from build123d import *

# Parameters (mm, degrees)
SKETCH011_W     = 40
SKETCH011_H     = 30
PAD003_DEPTH    = 10
CHAMFER_SIZE    = 3
PAD_DEPTH       = 17
POCKET_DEPTH    = 5
POCKET001_DEPTH = 4
POCKET002_DEPTH = 40.001
POCKET003_DEPTH = 40.001
PAD001_DEPTH    = 58
PAD002_DEPTH    = 8
POCKET004_DEPTH = 5
SKETCH010_R     = 3.1
POCKET005_DEPTH = 8.001
SKETCH005_R     = 3.4
POCKET006_DEPTH = 41.001
SKETCH012_R     = 8.1
POCKET007_DEPTH = 58.001
POCKET008_DEPTH = 57.5


with BuildPart() as inner_part:
    # Sketch011 → Pad003 (new body)
    with BuildSketch(Plane.XZ.offset(3.5)):
        with Locations((25, 30)):
            Rectangle(SKETCH011_W, SKETCH011_H)
    extrude(amount=PAD003_DEPTH)

    # Chamfer
    chamfer_edges = [inner_part.edges().sort_by_distance(p)[0] for p in [
        (25, -3.5, 45),
        (25, -13.5, 45),
    ]]
    chamfer(chamfer_edges, length=CHAMFER_SIZE)


with BuildPart() as rod_guide_slot:
    # Sketch → Pad (new body)
    with BuildSketch(Plane.XZ):
        Polygon((0, 0), (0, 13.079746), (-5, 21.74), (-5, 39.8), (0, 39.8), (0, 58), (40, 58), (40, 45), (31.339746, 30), (40, 15), (40, 0), align=None)
    extrude(amount=PAD_DEPTH)

    # Sketch001 → Pocket (cut)
    with BuildSketch(Plane(origin=(-5, 0, 0), x_dir=(0, 0, -1), z_dir=(-1, 0, 0))):
        Polygon((-34.892523, 17), (-39.8, 8.5), (-34.892523, 0), (-42.892523, 0), (-42.892523, 17), align=None)
    extrude(amount=-POCKET_DEPTH, mode=Mode.SUBTRACT)

    # Sketch002 → Pocket001 (cut)
    with BuildSketch(Plane(origin=(-5, 0, 0), x_dir=(0, 0, -1), z_dir=(-1, 0, 0))):
        Polygon((-35.89, 8.5), (-32.945, 13.60089), (-27.055, 13.60089), (-24.11, 8.5), (-27.055, 3.39911), (-32.945, 3.39911), align=None)
    extrude(amount=-POCKET001_DEPTH, mode=Mode.SUBTRACT)

    # Sketch003 → Pocket002 (cut, through all)
    with BuildSketch(Plane(origin=(0, 0, 0), x_dir=(0, 0, -1), z_dir=(-1, 0, 0))):
        with BuildLine():
            Line((-55.51292, 9.75), (-55.51292, 7.25))
            Line((-55.51292, 7.25), (-53.88146, 5.61854))
            ThreePointArc((-53.88146, 5.61854), (-46.925, 8.5), (-53.88146, 11.38146))
            Line((-55.51292, 9.75), (-53.88146, 11.38146))
        make_face()
    extrude(amount=-POCKET002_DEPTH, mode=Mode.SUBTRACT)

    # Sketch004 → Pocket003 (cut, through all)
    with BuildSketch(Plane(origin=(0, 0, 0), x_dir=(0, 0, -1), z_dir=(-1, 0, 0))):
        with BuildLine():
            Line((-10.51292, 9.75), (-10.51292, 7.25))
            Line((-10.51292, 7.25), (-8.88146, 5.61854))
            ThreePointArc((-8.88146, 5.61854), (-1.925, 8.5), (-8.88146, 11.38146))
            Line((-10.51292, 9.75), (-8.88146, 11.38146))
        make_face()
    extrude(amount=-POCKET003_DEPTH, mode=Mode.SUBTRACT)

    # Sketch006 → Pad001 (new body)
    with BuildSketch(Plane(origin=(0, 0, 0), x_dir=(1, 0, 0), z_dir=(0, 0, -1))):
        with BuildLine():
            Line((4, 23.5), (4, 17))
            Line((4, 17), (26, 17))
            Line((26, 23.5), (26, 17))
            ThreePointArc((26, 23.5), (15, 34.5), (4, 23.5))
        make_face()
    extrude(amount=-PAD001_DEPTH)

    # Sketch007 → Pad002 (new body)
    with BuildSketch(Plane(origin=(0, 0, 0), x_dir=(1, 0, 0), z_dir=(0, 0, -1))):
        Polygon((25.63, 17), (25.63, 26.32), (28, 30.43), (36, 30.43), (40, 23.5), (40, 17), align=None)
    extrude(amount=-PAD002_DEPTH)

    # Sketch009 → Pocket004 (cut)
    with BuildSketch(Plane(origin=(0, 0, 8), x_dir=(-1, 0, 0), z_dir=(0, 0, 1))):
        Polygon((-36.601482, 23.5), (-34.300741, 27.485), (-29.699259, 27.485), (-27.398518, 23.5), (-29.699259, 19.515), (-34.300741, 19.515), align=None)
    extrude(amount=-POCKET004_DEPTH, mode=Mode.SUBTRACT)

    # Sketch010 → Pocket005 (cut, through all)
    with BuildSketch(Plane(origin=(0, 0, 8), x_dir=(-1, 0, 0), z_dir=(0, 0, 1))):
        with Locations((-32, 23.5)):
            Circle(SKETCH010_R)
    extrude(amount=-POCKET005_DEPTH, mode=Mode.SUBTRACT)

    # Cut001: cut inner-part
    add(inner_part.part, mode=Mode.SUBTRACT)

    # Sketch005 → Pocket006 (cut, through all)
    with BuildSketch(Plane(origin=(-1, 0, 0), x_dir=(0, -1, 0), z_dir=(-1, 0, 0))):
        with Locations((8.5, 30)):
            Circle(SKETCH005_R)
    extrude(amount=-POCKET006_DEPTH, mode=Mode.SUBTRACT)

    # Sketch012 → Pocket007 (cut, through all)
    with BuildSketch(Plane.XY.offset(58)):
        with Locations((15, -23.5)):
            Circle(SKETCH012_R)
    extrude(amount=-POCKET007_DEPTH, mode=Mode.SUBTRACT)

    # Sketch013 → Pocket008 (cut)
    with BuildSketch(Plane.XY.offset(58)):
        Polygon((22.127646, -25.72736), (25.627646, -26.864579), (25.627646, -27.914579), (22.127646, -26.77736), align=None)
    extrude(amount=-POCKET008_DEPTH, mode=Mode.SUBTRACT)


solid = rod_guide_slot.part
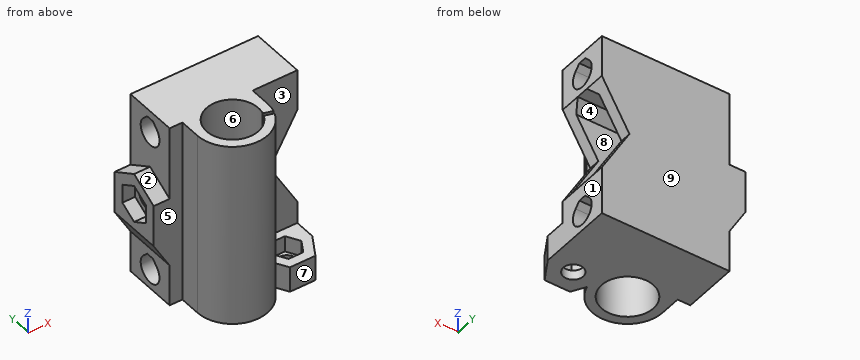
Could you check a few things on this model? Use its own coordinates, in mm. Face numbers are marked on the shaded views. A direction names the side the tool comes from. Round coordinates to 2 decimals unless told otherwise and drop trailing zeros. Write each loop counter-clockwise with the first axis right and the second up, starting at its lowest first coordinate (ties: lowest second). Pieces come first, ordered by that corner, then holes. Notation, with made-up numbers: (28, 45) - (82, 45) arc R28 ccw to (82, 66) - close; hole circle Ø2 at (-35.75, -7.75). An arc over 180 degrees is marked (long way). Use a Markdown table: item, result.
Q1. I want a section at C-C (z = 51). List the corners of the cut face in (x, y) for me (3 decimals), plus the area to 3 significant figures.
Output values:
| item | result |
|---|---|
| outline | (0, -17) - (4, -17) - (4, -23.5) arc R11 ccw to (25.143, -27.757) - (22.372, -26.857) arc R8.1 cw (long way) to (22.729, -25.923) - (25.487, -26.819) arc R11 ccw to (26, -23.5) - (26, -17) - (40, -17) - (40, -12.575) - (0, -12.575) - close; (0, -4.425) - (40, -4.425) - (40, 0) - (0, 0) - close |
| area | 478 mm2 |
Q2. I want a section at B-B (x = 30.5). List the corners of the cut face in (y, z) for me (3 decimals), plus the area to 3 significant figures.
Output values:
| item | result |
|---|---|
| outline | (-30.43, 0) - (-26.213, 0) - (-26.213, 3) - (-27.485, 3) - (-27.485, 8) - (-30.43, 8) - close; (-20.787, 0) - (0, 0) - (0, 58) - (-17, 58) - (-17, 8) - (-19.515, 8) - (-19.515, 3) - (-20.787, 3) - close; hole (-13.5, 15) - (-3.5, 15) - (-3.5, 42) - (-6.5, 45) - (-10.5, 45) - (-13.5, 42) - close; hole (-11.381, 8.881) arc R4.075 ccw (long way) to (-5.619, 8.881) - (-7.25, 10.513) - (-9.75, 10.513) - close; hole (-11.381, 53.881) arc R4.075 ccw (long way) to (-5.619, 53.881) - (-7.25, 55.513) - (-9.75, 55.513) - close |
| area | 638 mm2 |
Q3. I want a section at D-D (x = 14). List the corners of the cut face in (y, z) for me (3 decimals), plus the area to 3 significant figures.
Output values:
| item | result |
|---|---|
| outline | (-34.454, 0) - (-31.538, 0) - (-31.538, 58) - (-34.454, 58) - close; (-15.462, 0) - (0, 0) - (0, 58) - (-15.462, 58) - close; hole (-13.5, 15) - (-3.5, 15) - (-3.5, 42) - (-6.5, 45) - (-10.5, 45) - (-13.5, 42) - close; hole (-11.381, 8.881) arc R4.075 ccw (long way) to (-5.619, 8.881) - (-7.25, 10.513) - (-9.75, 10.513) - close; hole (-11.381, 53.881) arc R4.075 ccw (long way) to (-5.619, 53.881) - (-7.25, 55.513) - (-9.75, 55.513) - close |
| area | 667 mm2 |
Q4. I want a section at A-A (z = 6). List the corners of the cut face in (x, y) for me (3 decimals).
Output values:
| item | result |
|---|---|
| outline | (0, -17) - (4, -17) - (4, -23.5) arc R11 ccw to (25.143, -27.757) - (22.372, -26.857) arc R8.1 cw (long way) to (22.729, -25.923) - (25.487, -26.819) arc R11 ccw to (25.632, -26.323) - (28, -30.43) - (36, -30.43) - (40, -23.5) - (40, -12.575) - (0, -12.575) - close; (0, -4.425) - (40, -4.425) - (40, 0) - (0, 0) - close; hole (27.399, -23.5) - (29.699, -27.485) - (34.301, -27.485) - (36.601, -23.5) - (34.301, -19.515) - (29.699, -19.515) - close |
Q5. Please list where these lines run through material, in increasing order: L1, parallel to Y at x = 15, z = 37; L2, parallel to X at y = -23.5, z = 1.5; L3, parallel to Y at x = 8, z = 37.
Output values:
| item | result |
|---|---|
| L1 | -34.5 to -31.6, -15.4 to -13.5, -3.5 to 0 |
| L2 | 4 to 6.9, 23.1 to 28.9, 35.1 to 40 |
| L3 | -31.99 to -27.58, -19.42 to -13.5, -3.5 to 0 |
Q6. For the marked faces 1, 2, 3, 4 and 5, which set-ups out of +Z, -Z, +X, -X, +Y, -Y let a thin tool reach every point of the face, with its end or its side?
Output values:
| item | result |
|---|---|
| face 1 | +Z, -Z, +X, +Y, -Y |
| face 2 | +Z, -X, -Y |
| face 3 | +Z, +X, -Y |
| face 4 | +X |
| face 5 | +Z, -Z, -X, -Y |
Q7. For pin 1 (6.5 mm diameter, centred on x = 35, y = -20.5, fed in from +Z); pin 2 (5 mm diameter, centred on y = -6.5, z = 31.5, fed in from +X); pin 3 (12 mm diameter, centred on y = -28, z = 33.5, fed in from -X); pin 4 (13 mm diameter, centred on x = 15, y = -23.5, fed in from +Z), each with a flat end and sliding along its axis, tell me the tip position at first contact or that it passes through.
Output values:
| item | result |
|---|---|
| pin 1 | z = 8 |
| pin 2 | x = 5 |
| pin 3 | x = 4 |
| pin 4 | through |
Q8. Thinking about a two-plate mould opening in Y: for the marked faces 6, 7, 8 and 9, which applies, released by +Y, released by -Y, zero draft, split by the parting line, or undercut?
Output values:
| item | result |
|---|---|
| face 6 | undercut |
| face 7 | released by -Y |
| face 8 | undercut |
| face 9 | released by +Y |
